from build123d import *

# Parameters (mm, degrees)
SKETCH1_W           = 36.576
SKETCH1_H           = 36.576
BOSS_EXTRUDE1_DEPTH = 2.54
SKETCH2_R           = 1.5875
BOSS_EXTRUDE2_DEPTH = 25.4
CUT_EXTRUDE4_DEPTH  = 3.54
SKETCH4_R           = 8.001
BOSS_EXTRUDE3_DEPTH = 1.016
SKETCH5_R           = 2.49555
BOSS_EXTRUDE4_DEPTH = 19.05
SKETCH6_R           = 18.161
BOSS_EXTRUDE5_DEPTH = 20.828


with BuildPart() as part:
    # Sketch1 → Boss-Extrude1 (new body)
    with BuildSketch(Plane.XY):
        with Locations((17.649916168, -17.343808383)):
            Rectangle(SKETCH1_W, SKETCH1_H)
    extrude(amount=BOSS_EXTRUDE1_DEPTH)

    # Sketch2 → Boss-Extrude2 (add)
    with BuildSketch(Plane.XY.offset(2.54)):
        with Locations((33.143916168, -1.849808383)):
            Circle(SKETCH2_R)
        with Locations((2.155916168, -32.837808383)):
            Circle(SKETCH2_R)
    extrude(amount=BOSS_EXTRUDE2_DEPTH)

    # Sketch3 → Cut-Extrude4 (cut, through all)
    with BuildSketch(Plane.XY.offset(2.54)):
        with BuildLine():
            Line((-0.638083832, 0.944191617), (-0.638083832, -17.343808383))
            Line((-0.638083832, -17.343808383), (-0.511083832, -17.343808383))
            ThreePointArc((-0.511083832, -17.343808383), (4.808149915, -4.50204213), (17.649916168, 0.817191617))
            Line((17.649916168, 0.817191617), (17.649916168, 0.944191617))
            Line((17.649916168, 0.944191617), (-0.638083832, 0.944191617))
        make_face()
        with BuildLine():
            Line((35.937916168, -35.631808383), (17.649916168, -35.631808383))
            Line((17.649916168, -35.631808383), (17.649916168, -35.504808383))
            ThreePointArc((17.649916168, -35.504808383), (30.491682421, -30.185574636), (35.810916168, -17.343808383))
            Line((35.810916168, -17.343808383), (35.937916168, -17.343808383))
            Line((35.937916168, -17.343808383), (35.937916168, -35.631808383))
        make_face()
    extrude(amount=-CUT_EXTRUDE4_DEPTH, mode=Mode.SUBTRACT)

    # Sketch4 → Boss-Extrude3 (add)
    with BuildSketch(Plane(origin=(0, 0, 0), x_dir=(-1, 0, 0), z_dir=(0, 0, -1))):
        with Locations((-17.649916168, -17.343808383)):
            Circle(SKETCH4_R)
    extrude(amount=BOSS_EXTRUDE3_DEPTH)

    # Sketch5 → Boss-Extrude4 (add)
    with BuildSketch(Plane(origin=(0, 0, -1.016), x_dir=(-1, 0, 0), z_dir=(0, 0, -1))):
        with Locations((-17.649916168, -17.343808383)):
            Circle(SKETCH5_R)
    extrude(amount=BOSS_EXTRUDE4_DEPTH)

    # Sketch6 → Boss-Extrude5 (add)
    with BuildSketch(Plane.XY.offset(2.54)):
        with Locations((17.649916168, -17.343808383)):
            Circle(SKETCH6_R)
    extrude(amount=BOSS_EXTRUDE5_DEPTH)


solid = part.part
Check sheet for the modelled part. Datum: model origin and axes. Units: mm. A direction names the side the tool comes from. Round coordinates to 2 decimals unless told otherwise and drop trailing zeros. Order: outer loops, then holes, each group sorted by start corner. A loop starts at its lowest first (then second) coordinate and runs counter-clockwise, first axis right, second up. Notation, with made-up numbers: M 65.5,27 L 81.5,27 A29 ccw 81.5,63 Z; hole C 3,46.5 d1. An arc over 180 degrees is marked long. One line per item, written item: value. Start each with the question number.
1. Section check B-B on y = -6. Enter the section's corners in (x, z), and give its area (3 significant figures).
2. Release check for a two-part mould opening along Y. For faces 1 (the cylindrical face through (3.01, -31.5, 15.06)), 2 (the flat face through (35.938, -8, 1)), 3 (the flat face through (8, -35.632, 1)) record: released by +Y, released by -Y, zero draft, split by the parting line, or undercut.
3. Access from +Z, -Z, +X, -X, +Y, -Y to the whole of each face (thin tool, end or side, straight path). Record for faces 4 (the flat face through (31, -3, 2.54)), 5 (the cylindrical face through (19.384, -25.155, -0.501)), 6 (the flat face through (27, 0.944, 1)).
4. Section check C-C on z = -3. Enter the section's corners in (x, y).
5. Section check D-D on z = 22. Enter the section's corners in (x, y) (1 decimal), and give its area (3 significant figures).
6. Scan lines: line 1 along Z through (x, y) = (2.5, -20.5); line 2 along Z through (x, y) = (17.5, -24.5); line 3 along Y through (x, z) = (17.5, 15). Record each from-to range of solid material in increasing order.
7. Gauge pin test, flat ends, axial feed: P1, Ø2, axis at x = 21.5, y = -27.5, coming from the +Z side; P2, Ø4, axis at x = 13, z = 9, coming from the +Y side; P3, Ø2, axis at x = 23, z = 15, coming from the +Y side. Record the tip position at first contact, or that the pin passes through.
8. Section check A-A on x = 8. Enter the section's corners in (y, z), and give its area (3 significant figures).
Results found:
1. outline: M 3.47,0 L 35.94,0 L 35.94,2.54 L 31.83,2.54 L 31.83,23.37 L 3.47,23.37 Z
1. area: 673 mm^2
2. face 1: undercut
2. face 2: zero draft
2. face 3: released by -Y
3. face 4: +Z
3. face 5: -Z
3. face 6: +Z, -Z, +X, -X, +Y
4. outline: C 17.65,-17.34 d4.99
5. outline: C 17.6,-17.3 d36.3; C 2.2,-32.8 d3.2; C 33.1,-1.8 d3.2
5. area: 1,050 mm^2
6. line 1: 0 to 23.37
6. line 2: -1.02 to 23.37
6. line 3: -35.5 to 0.82
7. P1: z = 23.37
7. P2: y = 0.62
7. P3: y = 0.29
8. outline: M -35.63,0 L -1.96,0 L -1.96,23.37 L -32.73,23.37 L -32.73,2.54 L -35.63,2.54 Z
8. area: 726 mm^2
